```python
from build123d import *

# Parameters (mm, degrees)
BOSS_EXTRUDE1_DEPTH = 11
CHAMFER1_SIZE       = 1


with BuildPart() as part:
    # Sketch1 → Revolve1 (revolve)
    with BuildSketch(Plane.XY, mode=Mode.PRIVATE) as revolve1_sk:
        Polygon((3.276548208, 0), (6.5, 0), (6.5, 7), (7.5, 8), (3.276548208, 8), align=None)
    revolve(revolve1_sk.sketch.rotate(Axis((0, 18.90634256, 0), (0, -1, 0)), 90), axis=Axis((0, 18.90634256, 0), (0, -1, 0)))

    # Sketch2 → Boss-Extrude1 (add)
    with BuildSketch(Plane(origin=(0, 8, 0), x_dir=(1, 0, 0), z_dir=(0, 1, 0))):
        Polygon((8.082903769, 0), (4.041451884, 7), (-4.041451884, 7), (-8.082903769, 0), (-4.041451884, -7), (4.041451884, -7), align=None)
    extrude(amount=BOSS_EXTRUDE1_DEPTH)

    # Sketch3 → Revolve3 (revolve)
    with BuildSketch(Plane.XY, mode=Mode.PRIVATE) as revolve3_sk:
        Polygon((5.5, 19), (5.5, 23), (3.657937283, 23), (3.657937283, 25), (5.5, 25), (5.5, 26), (1.142283078, 26), (1.142283078, 19), align=None)
    revolve(revolve3_sk.sketch.rotate(Axis((0, 22.925153464, 0), (0, -1, 0)), 90), axis=Axis((0, 22.925153464, 0), (0, -1, 0)))

    # Chamfer1
    chamfer1_edges = [part.edges().sort_by_distance(p)[0] for p in [
        (0, 0, -6.5),
    ]]
    chamfer(chamfer1_edges, length=CHAMFER1_SIZE)


solid = part.part
```
Build history of the part. All positions in model axes, mm. A direction names the side the tool comes from. Round coordinates to 2 decimals unless told otherwise and drop trailing zeros. Write each loop counter-clockwise with the first axis right and the second up, starting at its lowest first coordinate (ties: lowest second). Pieces come first, ordered by that corner, then holes.
1) Band-saw the part on C-C, the plane y = 11.5. List the corners of the cut face in (x, z), and give its area (3 significant figures).
2) 3-axis set-ups, long thin cutter, end or side, ignore diameter. For faces 4 (the flat face through (0, 19, 0)), 5 (the flat face through (-3.9, 8, -6.6)), 6 (the cylindrical face through (3.245, 24.014, 1.688)): which of +Z, -Z, +X, -X, +Y, -Y reach the whole face in a straight line?
3) Band-saw the part on A-A, the plane y = 3. List the corners of the cut face in (x, z), and give its area (3 significant figures).
4) Pin check, flat tips, straight feed: pin 1 (1 mm diameter, centred on x = 2, z = -1, fed in from -Y); pin 2 (2 mm diameter, centred on y = 4.5, z = 4, fed in from +X); pin 3 (4 mm diameter, centred on x = 4.5, y = 11.5, fed in from -Z). Stop position of each tip, or through.
5) Mould opens along Y. For faces 1 (the flat face through (1, 23, 4)), 2 (the flat face through (6.09, 13.42, -3.45)), 3 (the flat face through (-3.9, 8, 6.7)) say: +Y half, -Y half, draft (parallel to the pull), parting line (faces both ways), or undercut.
6) Band-saw the part on D-D, the plane y = 22.5. List the corners of the cut face in (x, z).
7) Drill centre lines: probe 1 along X at (y, z) = (23.5, 0); probe 2 along X at (y, z) = (6.25, 0); probe 3 along Y at (x, z) = (-2.25, -1.5). Where is each one in solid material? Low to high.
Ans:
1. outline: (-8.08, 0) - (-4.04, -7) - (4.04, -7) - (8.08, 0) - (4.04, 7) - (-4.04, 7) - close
1. area: 170 mm2
2. face 4: +Y
2. face 5: -Z, -X, -Y
2. face 6: none
3. outline: circle Ø13 at (0, 0); hole circle Ø6.55 at (0, 0)
3. area: 99.0 mm2
4. pin 1: stops at y = 8
4. pin 2: stops at x = 5.77
4. pin 3: stops at z = -7
5. face 1: undercut
5. face 2: draft
5. face 3: -Y half
6. outline: circle Ø11 at (0, 0); hole circle Ø2.28 at (0, 0)
7. probe 1: x = -3.66 to -1.14, 1.14 to 3.66
7. probe 2: x = -6.5 to -3.28, 3.28 to 6.5
7. probe 3: y = 8 to 26
